Model file for the job. Use its own axes, mm. Face numbers are marked on the shaded views. Give positions to 0.01 mm unless a question says otherwise; leave off trailing zeros. Loops run counter-clockwise (first coordinate to the right, second up) from the corner with the lowest first, then second, coordinate; pieces in that order, holes last. Notation, with made-up numbers: (-25.75, 33) - (11.25, 33) arc R19 cw to (11.25, 44) - close; hole circle Ø9 at (-32.5, 70.25). An arc over 180 degrees is marked (long way). Answer as CSV lines item,"result". Start each with the question number.
Item 1: Pull direction Z, two halves, no side cores. Call the marked faces 1, 2, 3 and 4: pulls with the +Z half, pulls with the -Z half, needs draft (parallel to the pull), parting line crosses it, or undercut.
Item 2: Saw through at D-D on y = 0. Give the cut face in (x, z) (3 decimals), plus the area to 3 significant figures.
Item 3: Saw through at A-A on y = -21. Give the cut face in (x, z) (3 decimals).
Item 4: Saw through at B-B on z = 43.5. Give the cut face in (x, y).
Item 5: Saw through at C-C on x = 47.5. Give the cut face in (y, z) (3 decimals), plus the area to 3 significant figures.
Item 6: Pin check, flat tips, straight feed: pin 1 (5 mm diameter, centred on y = 46, z = 4, fed in from +X); pin 2 (12 mm diameter, centred on y = -18, z = 72, fed in from +X); pin 3 (6 mm diameter, centred on x = 25.5, z = 86, fed in from +Y). Stop position of each tip, or through.
Item 7: Drill centre lines: L1, parallel to Z at x = -33.5, y = -44 (3 decimals); L2, parallel to X at y = 0, z = 33.5. Where is each one in solid material? Low to high. Write a range as from..to.
Autodesk Inventor part; units mm, degrees
ref_plane "YZ Plane" through (0, 0, 0) normal (1, 0, 0) x (0, 1, 0)
ref_plane "XZ Plane" through (0, 0, 0) normal (0, 1, 0) x (-1, 0, 0)
ref_plane "XY Plane" through (0, 0, 0) normal (0, 0, 1) x (1, 0, 0)
sketch "Sketch1" plane through (0, 0, 0) normal (0, 0, 1) x (1, 0, 0)
  circle A0 centre (0, 0) radius 31.75
  circle A1 centre (0, 0) radius 63.5
  circle A2 centre (0, 0) radius 69.85
  line L0 (0, 0) -> (0, 69.85)
  line L1 (0, 0) -> (-60.4919, 34.925)
  line L2 (0, 0) -> (-60.4919, -34.925)
  line L3 (0, 0) -> (0, -69.85)
  line L4 (0, 0) -> (60.4919, -34.925)
  line L5 (0, 0) -> (60.4919, 34.925)
  point P0 (54.9926, 31.75)
  point P1 (27.4963, 15.875)
  point P2 (27.4963, -15.875)
  point P3 (54.9926, -31.75)
  point P4 (0, -63.5)
  point P5 (0, -31.75)
  point P6 (-27.4963, -15.875)
  point P7 (-54.9926, -31.75)
  point P8 (-54.9926, 31.75)
  point P9 (-27.4963, 15.875)
  point P10 (0, 31.75)
  point P11 (0, 63.5)
  dimension "d16" = 139.7
  dimension "d5" = 360
  dimension "d14" = 127
  dimension "d15" = 63.5
extrude "Extrusion1" add sketch "Sketch1" along normal blind 127 contours L5 A2 L4 A1 | A1 L0 A2 L5 | L4 A2 L3 A1 | A1 L1 A2 L0 | L3 A2 L2 A1 | A1 L2 A2 L1
extrude "Extrusion2" add sketch "Sketch1" along normal blind 6.35 contours A0 L5 A1 L4 | A0 L1 A1 L0 | L3 A1 L2 A0
sketch "Sketch2" plane through (0, 0, 127) normal (0, 0, 1) x (1, 0, 0)
  arc A0 (54.9926, 31.75) -> (0, 63.5) centre (0, 0) ccw
  circle A1 centre (0, 0) radius 63.5
  point P0 (54.9926, 31.75)
extrude "Extrusion3" add sketch "Sketch2" against normal blind 3.175
properties part number "Powder Canister"
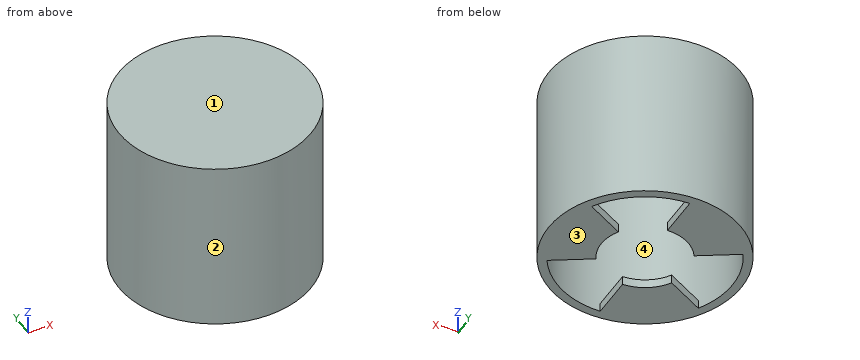
Responses:
1,face 1,"pulls with the +Z half"
1,face 2,"needs draft"
1,face 3,"pulls with the -Z half"
1,face 4,"undercut"
2,outline,"(-69.85, 0) - (-63.5, 0) - (-63.5, 123.825) - (63.5, 123.825) - (63.5, 6.35) - (31.75, 6.35) - (31.75, 0) - (69.85, 0) - (69.85, 127) - (-69.85, 127) - close"
2,area,"2,220 mm2"
3,outline,"(-66.618, 0) - (-59.927, 0) - (-59.927, 123.825) - (59.927, 123.825) - (59.927, 6.35) - (36.373, 6.35) - (36.373, 0) - (66.618, 0) - (66.618, 127) - (-66.618, 127) - close; (-36.373, 0) - (-23.813, 0) - (-23.813, 6.35) - (-36.373, 6.35) - close"
4,outline,"circle Ø139.7 at (0, 0); hole circle Ø127 at (0, 0)"
5,outline,"(-51.213, 0) - (-42.143, 0) - (-42.143, 123.825) - (42.143, 123.825) - (42.143, 0) - (51.213, 0) - (51.213, 127) - (-51.213, 127) - close; (-27.424, 0) - (27.424, 0) - (27.424, 6.35) - (-27.424, 6.35) - close"
5,area,"2,920 mm2"
6,pin 1,"x = 54.65"
6,pin 2,"x = 68.81"
6,pin 3,"y = 66.13"
7,L1,"0..6.35, 123.825..127"
7,L2,"-69.85..-63.5, 63.5..69.85"
